Autodesk Inventor part; units mm, degrees
ref_plane "YZ Plane" through (0, 0, 0) normal (1, 0, 0) x (0, 1, 0)
ref_plane "XZ Plane" through (0, 0, 0) normal (0, 1, 0) x (-1, 0, 0)
ref_plane "XY Plane" through (0, 0, 0) normal (0, 0, 1) x (1, 0, 0)
sketch "Sketch1" plane through (0, 0, 0) normal (0, 0, 1) x (1, 0, 0)
  line L0 (0, 0) -> (120.65, 0)
  line L1 (120.65, 0) -> (120.65, 113.919)
  line L2 (0, 113.919) -> (0, 0)
  circle A0 centre (11.2141, 60.325) radius 1.9431
  circle A1 centre (60.325, 11.2141) radius 1.9431
  circle A2 centre (109.4359, 60.325) radius 1.9431
  circle A3 centre (60.325, 109.4359) radius 1.9431
  line L3 (60.325, 113.919) -> (120.65, 113.919)
  line L4 (60.325, 113.919) -> (0, 113.919)
  line L5 (60.0329, 51.689) -> (69.9389, 51.689)
  line L6 (69.9389, 51.689) -> (69.9389, 43.18)
  line L7 (69.9389, 43.18) -> (60.0329, 43.18)
  line L8 (60.0329, 43.18) -> (60.0329, 51.689)
  point P0 (60.325, 60.325)
  dimension "d10" = 3.8862
  dimension "d13" = 360
  dimension "d34" = 9.906
  dimension "d35" = 8.509
extrude "Extrusion4" add sketch "Sketch1" along normal blind 25.4
properties part number "speakerfront2"
Can you work these out from the model? Positions are in its coordinate system, mm. A direction names the side the tool comes from. Coordinates: 2 decimals unless noted, no trailing zeros. Loops run counter-clockwise (first coordinate to the right, second up) from the corner with the lowest first, then second, coordinate; pieces in that order, holes last. Notation, with made-up numbers: (-23.75, 53.25) - (-15.75, 53.25) arc R26 ccw to (-15.75, 68.25) - close; hole circle Ø10 at (-24, 30.25). An arc over 180 degrees is marked (long way). Use a Markdown table: item, result.
Item 1: I want a section at B-B on y = 49. Please give me the cut outline in (x, z).
Numbers:
| item | result |
|---|---|
| outline | (0, 0) - (60.03, 0) - (60.03, 25.4) - (0, 25.4) - close; (69.94, 0) - (120.65, 0) - (120.65, 25.4) - (69.94, 25.4) - close |
Item 2: I want a section at A-A on x = 64. Please give me the cut outline in (y, z), and give its area (3 significant figures).
Numbers:
| item | result |
|---|---|
| outline | (0, 0) - (43.18, 0) - (43.18, 25.4) - (0, 25.4) - close; (51.69, 0) - (113.92, 0) - (113.92, 25.4) - (51.69, 25.4) - close |
| area | 2,680 mm2 |
Item 3: We'd pull the mould along Y, two halves only. Please class faces 1 (the face through (61, 113.919, 13)), 2 (the face through (59, 58, 0)), 3 (the face through (65, 51.689, 13)): released by +Y, released by -Y, zero draft, split by the parting line, or undercut.
Numbers:
| item | result |
|---|---|
| face 1 | released by +Y |
| face 2 | zero draft |
| face 3 | undercut |
Item 4: If I drill on probe 1 along Y at (x, z) = (11.5, 15.75); probe 2 along Y at (x, z) = (61, 1.75); probe 3 along Y at (x, z) = (111, 14), over which ranges is the centre line in solid material (lowest first)? Write a range as from..to.
Numbers:
| item | result |
|---|---|
| probe 1 | y = 0..58.4, 62.25..113.92 |
| probe 2 | y = 0..9.39, 13.04..43.18, 51.69..107.61, 111.26..113.92 |
| probe 3 | y = 0..59.17, 61.48..113.92 |
Item 5: For faces 4 (the face through (59, 58, 25.4)), 5 (the face through (60.033, 47, 13)), which set-ups out of +Z, -Z, +X, -X, +Y, -Y let a thin tool reach every point of the face, with its end or its side?
Numbers:
| item | result |
|---|---|
| face 4 | +Z, +X, -X, +Y, -Y |
| face 5 | +Z, -Z |
